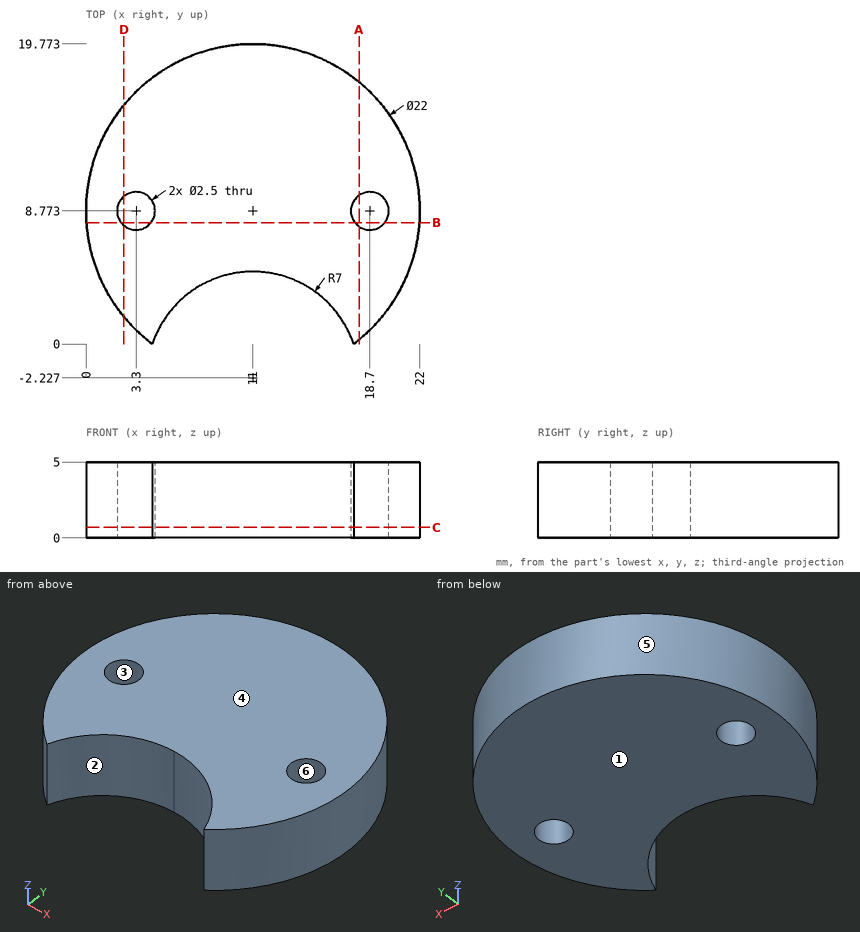
Geometry check sheet. Reference: drawing and pictorial views, mm from the part's lowest x, y, z. A direction names the side the tool comes from. Round coordinates to 2 decimals unless told otherwise and drop trailing zeros. Loops run counter-clockwise (first coordinate to the right, second up) from the corner with the lowest first, then second, coordinate; pieces in that order, holes last. Notation, with made-up numbers: (23, 20.25) -> (46, 20.25) arc R25 ccw to (46, 39.25) -> close; hole circle Ø11 at (-20, 59). An arc over 180 degrees is marked (long way). Answer as a JSON object with one key per item and string values.
Q1. Access from +Z, -Z, +X, -X, +Y, -Y to the whole of each face (thin tool, end or side, straight path). Record for the marked faces 1 and 2.
Data:
{"face 1": "-Z, +X, -X, +Y, -Y", "face 2": "+Z, -Z, -Y"}
Q2. Scan lines: line 1 (X direction, y = 8, z = 3.6); line 2 (Y direction, x = 18.7, z = 1.35); line 3 (X direction, y = 7.75, z = 4). Record each from-to range of solid material in increasing order. Write a range as from..to.
Data:
{"line 1": "x = 0.03..2.32, 4.28..17.72, 19.68..21.97", "line 2": "y = 0.92..7.52, 10.02..16.63", "line 3": "x = 0.05..2.58, 4.02..17.98, 19.42..21.95"}
Q3. Section check A-A (x = 18). Record the boundary of the cut face in (y, z), then the cut area to 3 significant figures.
Data:
{"outline": "(0.29, 0) -> (7.74, 0) -> (7.74, 5) -> (0.29, 5) -> close; (9.81, 0) -> (17.26, 0) -> (17.26, 5) -> (9.81, 5) -> close", "area": "74.5 mm2"}
Q4. Section check C-C (z = 0.7). Record the boundary of the cut face in (x, y), then the cut area to 3 significant figures.
Data:
{"outline": "(4.36, 0) arc R7 cw to (11, 4.77) arc R7 cw to (17.64, 0) arc R11 ccw (long way) to start; hole circle Ø2.5 at (3.3, 8.77); hole circle Ø2.5 at (18.7, 8.77)", "area": "304 mm2"}
Q5. Section check B-B (y = 8). Record the boundary of the cut face in (x, z).
Data:
{"outline": "(0.03, 0) -> (2.32, 0) -> (2.32, 5) -> (0.03, 5) -> close; (4.28, 0) -> (17.72, 0) -> (17.72, 5) -> (4.28, 5) -> close; (19.68, 0) -> (21.97, 0) -> (21.97, 5) -> (19.68, 5) -> close"}
Q6. Draft check along Y on the marked faces 3, 4, 5 and 6. Enter one of: pulls with the +Y half, pulls with the -Y half, needs draft (parallel to the pull), parting line crosses it, or undercut.
Data:
{"face 3": "undercut", "face 4": "needs draft", "face 5": "parting line crosses it", "face 6": "undercut"}
Q7. Section check D-D (x = 2.5). Record the boundary of the cut face in (y, z) (1 decimal), then the cut area to 3 significant figures.
Data:
{"outline": "(1.8, 0) -> (7.8, 0) -> (7.8, 5) -> (1.8, 5) -> close; (9.7, 0) -> (15.8, 0) -> (15.8, 5) -> (9.7, 5) -> close", "area": "60.2 mm2"}
Q8. Go/stop test with flat-tipped pins: P1, Ø3, axis at x = 8, z = 3.5, coming from the +Y side; P2, Ø3, axis at y = 11, z = 3.5, coming from the -X side; P3, Ø2, axis at y = 2.5, z = 2, coming from the -X side. Record where each tip stops, or that it passes through.
Data:
{"P1": "stops at y = 19.67", "P2": "stops at x = 0.02", "P3": "stops at x = 1.35"}
